Read the model definition and answer for the solid it produces. Units are mm, in the model's axes. A direction names the side the tool comes from. Give positions to 0.01 mm unless a question says otherwise; leave off trailing zeros. Order: outer loops, then holes, each group sorted by start corner. A loop starts at its lowest first (then second) coordinate and runs counter-clockwise, first axis right, second up.
Item 1: Find the intervals of material crossed by line 1 along Y through (x, z) = (6, 0.65); line 2 along Y through (x, z) = (1.5, 0.4), in increasing order.
Item 2: Which of the six approach directions +Z, -Z, +X, -X, +Y, -Y give full straight-line access (tool end or side, diameter ignored) to faces 1 (the face through (-10.7, 25.053, 0.5)), 2 (the face through (11.4, 25.053, 0.5)), 3 (the face through (-0.156, -23.093, 0.254)), 4 (the face through (0.6, 25.053, 0.5))?
Item 3: Given pin 1 Ø1.7 at (x, y) = (1.5, -25) entering from -Z; pin 2 Ø0.5 at (x, z) = (10, 0.5) entering from +Y; pin 3 Ø0.5 at (y, z) = (25.5, 0.5) entering from +X, each flat-ended and moving along its own axis, determine where each tip first touches the part or whether it passes through.
Item 4: A cutting plane is placed at A-A (z = 0.25). Write down the section's boundary in (x, y).
from build123d import *

# Parameters (mm, degrees)
SKETCH1_W               = 24
SKETCH1_H               = 51.6
BOSS_EXTRUDE1_DEPTH     = 1
SKETCH2_W               = 1.52454199
SKETCH2_H               = 0.68782272
BOSS_EXTRUDE2_DEPTH     = 1
CUT_EXTRUDE1_DEPTH      = 30.156315931
CUT_EXTRUDE1_DEPTH_BACK = 0.5


with BuildPart() as part:
    # Sketch1 → Boss-Extrude1 (new body)
    with BuildSketch(Plane.XY):
        with Locations((-0.014342532, -0.747058824)):
            Rectangle(SKETCH1_W, SKETCH1_H)
    extrude(amount=BOSS_EXTRUDE1_DEPTH)

    # Sketch2 → Boss-Extrude2 (add)
    with BuildSketch(Plane(origin=(0, 0, 0), x_dir=(-1, 0, 0), z_dir=(0, 0, -1))):
        with Locations((-10.081520714, 25.194355877)):
            Rectangle(SKETCH2_W, SKETCH2_H)
        with Locations((8.590054208, 25.199009148)):
            Rectangle(SKETCH2_W, SKETCH2_H)
    extrude(amount=-BOSS_EXTRUDE2_DEPTH)

    # Sketch3 → Cut-Extrude1 (cut, two sides: drawn at the far end of the back side and taken through both)
    with BuildSketch(Plane(origin=(0, 0, 0), x_dir=(-1, 0, 0), z_dir=(0, 0, -1)).offset(-CUT_EXTRUDE1_DEPTH_BACK)):
        with BuildLine():
            Line((-3.38328462, -26.547058824), (3.544014575, -26.547058824))
            ThreePointArc((3.544014575, -26.547058824), (0.080364977, -23.092635137), (-3.38328462, -26.547058824))
        make_face()
    extrude(amount=CUT_EXTRUDE1_DEPTH + CUT_EXTRUDE1_DEPTH_BACK, mode=Mode.SUBTRACT)


solid = part.part
Response values:
1. line 1: y = -26.55 to 25.05
1. line 2: y = -23.47 to 25.05
2. face 1: +Z, -Z, -X, +Y
2. face 2: +Z, -Z, +X, +Y
2. face 3: -Z, -Y
2. face 4: +Z, -Z, +Y
3. pin 1: stops at z = 0.5
3. pin 2: stops at y = 25.54
3. pin 3: stops at x = 10.84
4. outline: (-12.01, -26.55) - (-3.54, -26.55) arc R3.46 cw to (3.38, -26.55) - (11.99, -26.55) - (11.99, 25.05) - (10.84, 25.05) - (10.84, 25.54) - (9.32, 25.54) - (9.32, 25.05) - (-7.83, 25.05) - (-7.83, 25.54) - (-9.35, 25.54) - (-9.35, 25.05) - (-12.01, 25.05) - close
